from build123d import *

# Parameters (mm, degrees)
F1_DEPTH  = 26
F2_DEPTH  = 4
F3_W      = 90
F3_H      = 64
F4_DEPTH  = 2
F6_DEPTH  = 2
F7_R      = 2.5
F8_DEPTH  = 2
F9_R      = 2.5
F10_DEPTH = 2
F11_W     = 5
F11_H     = 50
F11_W_2   = 76
F11_H_2   = 5
F12_DEPTH = 22
F13_R     = 1
F14_DEPTH = 5
F15_R     = 11
F15_R_2   = 5
F16_DEPTH = 2
F17_DEPTH = 5
F19_W     = 20.16
F19_H     = 11.52
F19_R     = 3
F19_R_2   = 2
F20_DEPTH = 5
F19_W_2   = 66
F19_H_2   = 18
F19_R_3   = 1.8
F21_DEPTH = 3
F22_DEPTH = 3
F19_R_4   = 0.8
F23_DEPTH = 1.9
F24_DEPTH = 1.9
F25_DEPTH = 1.9


# Not quite as in the source:
# - a feature names something its author has since deleted; it is built from what else it names


with BuildPart() as f1:
    # F0 (on Top) → F1 (new body)
    with BuildSketch(Plane.XY):
        with BuildLine():
            Line((46, 35), (-46, 35))
            ThreePointArc((-46, 35), (-47.4142135624, 34.4142135624), (-48, 33))
            Line((-48, 33), (-48, -33))
            ThreePointArc((-48, -33), (-47.4142135624, -34.4142135624), (-46, -35))
            Line((-46, -35), (46, -35))
            ThreePointArc((46, -35), (47.4142135624, -34.4142135624), (48, -33))
            Line((48, -33), (48, 33))
            ThreePointArc((48, 33), (47.4142135624, 34.4142135624), (46, 35))
        make_face()
    extrude(amount=F1_DEPTH)


with BuildPart() as f2:
    # F2 (new): a face of the model
    f2_faces = [f1.part.faces().sort_by_distance(p)[0] for p in [
        (0, 0, 26),
    ]]
    extrude(f2_faces, amount=F2_DEPTH)

    # F5 (on face) → F6 (join)
    with BuildSketch(Plane.XY.offset(30)):
        with BuildLine():
            Line((45.25, 33), (-45.25, 33))
            ThreePointArc((-45.25, 33), (-45.7803300859, 32.7803300859), (-46, 32.25))
            Line((-46, 32.25), (-46, -32.25))
            ThreePointArc((-46, -32.25), (-45.7803300859, -32.7803300859), (-45.25, -33))
            Line((-45.25, -33), (45.25, -33))
            ThreePointArc((45.25, -33), (45.7803300859, -32.7803300859), (46, -32.25))
            Line((46, -32.25), (46, 32.25))
            ThreePointArc((46, 32.25), (45.7803300859, 32.7803300859), (45.25, 33))
        make_face()
        with BuildLine():
            ThreePointArc((-45.25, 32), (-45.1767766953, 32.1767766953), (-45, 32.25))
            Line((-45, 32.25), (45, 32.25))
            ThreePointArc((45, 32.25), (45.1767766953, 32.1767766953), (45.25, 32))
            Line((45.25, 32), (45.25, -32))
            ThreePointArc((45.25, -32), (45.1767766953, -32.1767766953), (45, -32.25))
            Line((45, -32.25), (-45, -32.25))
            ThreePointArc((-45, -32.25), (-45.1767766953, -32.1767766953), (-45.25, -32))
            Line((-45.25, -32), (-45.25, 32))
        make_face(mode=Mode.SUBTRACT)
    extrude(amount=F6_DEPTH)

    # F9 (on face) → F10 (cut)
    with BuildSketch(Plane.XY.offset(30)):
        with Locations((-41.75, -28.75)):
            Circle(F9_R)
        with Locations((-41.75, 28.75)):
            Circle(F9_R)
        with Locations((41.75, 28.75)):
            Circle(F9_R)
        with Locations((41.75, -28.75)):
            Circle(F9_R)
    extrude(amount=-F10_DEPTH, mode=Mode.SUBTRACT)


with BuildPart() as f1_1:
    add(f1.part)

    # F3 (on face) → F4 (cut)
    with BuildSketch(Plane.XY.offset(26)):
        with BuildLine():
            Line((45, 33), (-45, 33))
            ThreePointArc((-45, 33), (-45.7071067812, 32.7071067812), (-46, 32))
            Line((-46, 32), (-46, -32))
            ThreePointArc((-46, -32), (-45.7071067812, -32.7071067812), (-45, -33))
            Line((-45, -33), (45, -33))
            ThreePointArc((45, -33), (45.7071067812, -32.7071067812), (46, -32))
            Line((46, -32), (46, 32))
            ThreePointArc((46, 32), (45.7071067812, 32.7071067812), (45, 33))
        make_face()
        Rectangle(F3_W, F3_H, mode=Mode.SUBTRACT)
    extrude(amount=-F4_DEPTH, mode=Mode.SUBTRACT)

    # F7 (on face) → F8 (cut)
    with BuildSketch(Plane.XY.offset(26)):
        with Locations((-41.5, -28.5)):
            Circle(F7_R)
        with Locations((-41.4999984205, 28.5)):
            Circle(F7_R)
        with Locations((41.5, 28.5)):
            Circle(F7_R)
        with Locations((41.5, -28.5)):
            Circle(F7_R)
    extrude(amount=-F8_DEPTH, mode=Mode.SUBTRACT)

    # F11 (on face) → F12 (cut)
    with BuildSketch(Plane.XY.offset(26)):
        with Locations((-40.5, 0)):
            Rectangle(F11_W, F11_H)
        with Locations((0, -27.5)):
            Rectangle(F11_W_2, F11_H_2)
        Rectangle(F11_W_2, F11_H)
        with Locations((0, 27.5)):
            Rectangle(F11_W_2, F11_H_2)
        with Locations((40.5, 0)):
            Rectangle(F11_W, F11_H)
    extrude(amount=-F12_DEPTH, mode=Mode.SUBTRACT)

    # F13 (on face) → F14 (cut, through all)
    with BuildSketch(Plane.YZ.offset(48)):
        with Locations((7.9999985173, 14.5000000224)):
            Circle(F13_R)
        with Locations((7.9999985173, 11.5000000224)):
            Circle(F13_R)
        with Locations((10.9999985173, 11.5000000224)):
            Circle(F13_R)
        with Locations((10.9999985173, 14.5000000224)):
            Circle(F13_R)
        with Locations((13.9999985173, 14.5000000224)):
            Circle(F13_R)
        with Locations((13.9999985173, 11.5000000224)):
            Circle(F13_R)
    extrude(amount=-F14_DEPTH, mode=Mode.SUBTRACT)

    # F15 (on face) → F16 (cut)
    with BuildSketch(Plane(origin=(-48, 0, 0), x_dir=(0, -1, 0), z_dir=(-1, 0, 0))):
        with Locations((6.9999988191, 12.5000002682)):
            Circle(F15_R)
        with Locations((6.9999988191, 12.5000002682)):
            Circle(F15_R_2, mode=Mode.SUBTRACT)
    extrude(amount=-F16_DEPTH, mode=Mode.SUBTRACT)

    # F15 (on face) → F17 (cut, through all)
    with BuildSketch(Plane(origin=(-48, 0, 0), x_dir=(0, -1, 0), z_dir=(-1, 0, 0))):
        with Locations((6.9999988191, 12.5000002682)):
            Circle(F15_R_2)
    extrude(amount=-F17_DEPTH, mode=Mode.SUBTRACT)

    # F19 (on face) → F20 (cut, through all)
    with BuildSketch(Plane(origin=(0, -30, 0), x_dir=(-1, 0, 0), z_dir=(0, 1, 0))):
        with Locations((4.7299169147, 14.0678631142)):
            Rectangle(F19_W, F19_H)
        with Locations((28.8399169147, 14.0678631142)):
            Circle(F19_R)
        with Locations((-11.1500830853, 14.0678631142)):
            Circle(F19_R_2)
        with Locations((-17.7100830853, 14.0678631142)):
            Circle(F19_R_2)
        with Locations((-24.2600830853, 14.0678631142)):
            Circle(F19_R_2)
        with BuildLine():
            ThreePointArc((-30.8900830853, 11.0678631142), (-30.5971898665, 10.360756333), (-29.8900830853, 10.0678631142))
            Line((-29.8900830853, 10.0678631142), (-28.9900830853, 10.0678631142))
            ThreePointArc((-28.9900830853, 10.0678631142), (-28.2829763041, 10.360756333), (-27.9900830853, 11.0678631142))
            Line((-27.9900830853, 11.0678631142), (-27.9900830853, 17.0678631142))
            ThreePointArc((-27.9900830853, 17.0678631142), (-28.2829763041, 17.7749698954), (-28.9900830853, 18.0678631142))
            Line((-28.9900830853, 18.0678631142), (-29.8900830853, 18.0678631142))
            ThreePointArc((-29.8900830853, 18.0678631142), (-30.5971898665, 17.7749698954), (-30.8900830853, 17.0678631142))
            Line((-30.8900830853, 17.0678631142), (-30.8900830853, 11.0678631142))
        make_face()
    extrude(amount=-F20_DEPTH, mode=Mode.SUBTRACT)

    # F19 (on face) → F21 (cut)
    with BuildSketch(Plane(origin=(0, -30, 0), x_dir=(-1, 0, 0), z_dir=(0, 1, 0))):
        with Locations((-0.1600830853, 14.0678631142)):
            Rectangle(F19_W_2, F19_H_2)
        with Locations((-24.0000830853, 7.5678631142)):
            Circle(F19_R_3, mode=Mode.SUBTRACT)
        with BuildLine():
            Line((-28.9900830853, 10.0678631142), (-29.8900830853, 10.0678631142))
            ThreePointArc((-29.8900830853, 10.0678631142), (-30.5971898665, 10.360756333), (-30.8900830853, 11.0678631142))
            Line((-30.8900830853, 11.0678631142), (-30.8900830853, 17.0678631142))
            ThreePointArc((-30.8900830853, 17.0678631142), (-30.5971898665, 17.7749698954), (-29.8900830853, 18.0678631142))
            Line((-29.8900830853, 18.0678631142), (-28.9900830853, 18.0678631142))
            ThreePointArc((-28.9900830853, 18.0678631142), (-28.2829763041, 17.7749698954), (-27.9900830853, 17.0678631142))
            Line((-27.9900830853, 17.0678631142), (-27.9900830853, 11.0678631142))
            ThreePointArc((-27.9900830853, 11.0678631142), (-28.2829763041, 10.360756333), (-28.9900830853, 10.0678631142))
        make_face(mode=Mode.SUBTRACT)
        with Locations((-24.2600830853, 14.0678631142)):
            Circle(F19_R_2, mode=Mode.SUBTRACT)
        with Locations((-17.7100830853, 14.0678631142)):
            Circle(F19_R_2, mode=Mode.SUBTRACT)
        with Locations((-11.1500830853, 14.0678631142)):
            Circle(F19_R_2, mode=Mode.SUBTRACT)
        with Locations((30.1799169147, 7.5678631142)):
            Circle(F19_R_3, mode=Mode.SUBTRACT)
        with Locations((4.7299169147, 14.0678631142)):
            Rectangle(F19_W, F19_H, mode=Mode.SUBTRACT)
        with Locations((28.8399169147, 14.0678631142)):
            Circle(F19_R, mode=Mode.SUBTRACT)
        with Locations((30.1799169147, 20.5678631142)):
            Circle(F19_R_3, mode=Mode.SUBTRACT)
    extrude(amount=F21_DEPTH, mode=Mode.SUBTRACT)

    # F19 (on face) → F22 (cut)
    with BuildSketch(Plane(origin=(0, -30, 0), x_dir=(-1, 0, 0), z_dir=(0, 1, 0))):
        with Locations((-0.1600830853, 14.0678631142)):
            Rectangle(F19_W_2, F19_H_2)
        with Locations((-24.0000830853, 7.5678631142)):
            Circle(F19_R_3, mode=Mode.SUBTRACT)
        with BuildLine():
            Line((-28.9900830853, 10.0678631142), (-29.8900830853, 10.0678631142))
            ThreePointArc((-29.8900830853, 10.0678631142), (-30.5971898665, 10.360756333), (-30.8900830853, 11.0678631142))
            Line((-30.8900830853, 11.0678631142), (-30.8900830853, 17.0678631142))
            ThreePointArc((-30.8900830853, 17.0678631142), (-30.5971898665, 17.7749698954), (-29.8900830853, 18.0678631142))
            Line((-29.8900830853, 18.0678631142), (-28.9900830853, 18.0678631142))
            ThreePointArc((-28.9900830853, 18.0678631142), (-28.2829763041, 17.7749698954), (-27.9900830853, 17.0678631142))
            Line((-27.9900830853, 17.0678631142), (-27.9900830853, 11.0678631142))
            ThreePointArc((-27.9900830853, 11.0678631142), (-28.2829763041, 10.360756333), (-28.9900830853, 10.0678631142))
        make_face(mode=Mode.SUBTRACT)
        with Locations((-24.2600830853, 14.0678631142)):
            Circle(F19_R_2, mode=Mode.SUBTRACT)
        with Locations((-17.7100830853, 14.0678631142)):
            Circle(F19_R_2, mode=Mode.SUBTRACT)
        with Locations((-11.1500830853, 14.0678631142)):
            Circle(F19_R_2, mode=Mode.SUBTRACT)
        with Locations((30.1799169147, 7.5678631142)):
            Circle(F19_R_3, mode=Mode.SUBTRACT)
        with Locations((4.7299169147, 14.0678631142)):
            Rectangle(F19_W, F19_H, mode=Mode.SUBTRACT)
        with Locations((28.8399169147, 14.0678631142)):
            Circle(F19_R, mode=Mode.SUBTRACT)
        with Locations((30.1799169147, 20.5678631142)):
            Circle(F19_R_3, mode=Mode.SUBTRACT)
    extrude(amount=-F22_DEPTH, mode=Mode.SUBTRACT)

    # F19 (on face) → F23 (join)
    with BuildSketch(Plane(origin=(0, -30, 0), x_dir=(-1, 0, 0), z_dir=(0, 1, 0))):
        with Locations((30.1799169147, 20.5678631142)):
            Circle(F19_R_3)
        with Locations((30.1799169147, 20.5678631142)):
            Circle(F19_R_4, mode=Mode.SUBTRACT)
    extrude(amount=F23_DEPTH)

    # F19 (on face) → F24 (join)
    with BuildSketch(Plane(origin=(0, -30, 0), x_dir=(-1, 0, 0), z_dir=(0, 1, 0))):
        with Locations((30.1799169147, 7.5678631142)):
            Circle(F19_R_3)
        with Locations((30.1799169147, 7.5678631142)):
            Circle(F19_R_4, mode=Mode.SUBTRACT)
    extrude(amount=F24_DEPTH)

    # F19 (on face) → F25 (join)
    with BuildSketch(Plane(origin=(0, -30, 0), x_dir=(-1, 0, 0), z_dir=(0, 1, 0))):
        with Locations((-24.0000830853, 7.5678631142)):
            Circle(F19_R_3)
        with Locations((-24.0000830853, 7.5678631142)):
            Circle(F19_R_4, mode=Mode.SUBTRACT)
    extrude(amount=F25_DEPTH)


with BuildPart() as f27_1:
    # F27: copy of F2
    add(f2.part)


with BuildPart() as f29_1:
    # F29: copy of F2
    add(f2.part)


solid = f2.part
Geometry check sheet. Reference: the model listing, model coordinates, mm. A direction names the side the tool comes from. Round coordinates to 2 decimals unless told otherwise and drop trailing zeros. Loops run counter-clockwise (first coordinate to the right, second up) from the corner with the lowest first, then second, coordinate; pieces in that order, holes last.
Item 1: Gauge pin test, flat ends, axial feed: pin 1 (0.6 mm diameter, centred on y = 2.5, z = 31, fed in from -X); pin 2 (2.5 mm diameter, centred on x = -42.5, y = -29, fed in from +Z); pin 3 (1 mm diameter, centred on x = -3, z = 31, fed in from -Y). Record the tip position at first contact, or that the pin passes through.
Item 2: Access from +Z, -Z, +X, -X, +Y, -Y to the whole of each face (thin tool, end or side, straight path). Record for faces 4 (the flat face through (-46, 0, 31)), 5 (the flat face through (-1, -35, 28)), 6 (the flat face through (1, 33, 31)), 7 (the flat face through (46, 0, 31)), 8 (the cylindrical face through (43.09, 30.86, 29.01)).
Item 3: Cross-section at A-A on x = -38. Record the boundary of the cut face in (y, z), then the cut area to 3 significant figures.
Item 4: Thickness scan on line 1 (Y direction, x = 41.75, z = 28.9); line 2 (X direction, y = 14, z = 30.75); line 3 (Y direction, x = 28, z = 30.8). Record the ranges inside material, lowest first.
Item 5: Cross-section at C-C on x = 40.5. Record the boundary of the cut face in (y, z), then the cut area to 3 significant figures.
Item 6: Cross-section at B-B on y = 22. Record the boundary of the cut face in (x, z).
Item 7: Mould release check, pull along X, two halves, no side actions. Record for faces 1 (the cylindrical face through (-47.4, 34.43, 27.97)), 2 (the flat face through (1, -32.25, 31)), 3 (the flat face through (-1, 0, 26)): pulls with the +X half, pulls with the -X half, needs draft (parallel to the pull), parting line crosses it, or undercut.
Answer sheet:
1. pin 1: stops at x = -46
1. pin 2: stops at z = 28
1. pin 3: stops at y = -33
2. face 4: +Z, -X, +Y, -Y
2. face 5: +Z, -Z, +X, -X, -Y
2. face 6: +Z, +X, -X, +Y
2. face 7: +Z, +X, +Y, -Y
2. face 8: +Z
3. outline: (-35, 26) - (35, 26) - (35, 30) - (33, 30) - (33, 32) - (32.25, 32) - (32.25, 30) - (-32.25, 30) - (-32.25, 32) - (-33, 32) - (-33, 30) - (-35, 30) - close
3. area: 283 mm2
4. line 1: y = -35 to -31.25, -26.25 to 26.25, 31.25 to 35
4. line 2: x = -46 to -45.25, 45.25 to 46
4. line 3: y = -33 to -32.25, 32.25 to 33
5. outline: (-35, 26) - (35, 26) - (35, 30) - (33, 30) - (33, 32) - (32.25, 32) - (32.25, 30) - (30.92, 30) - (30.92, 28) - (26.58, 28) - (26.58, 30) - (-26.58, 30) - (-26.58, 28) - (-30.92, 28) - (-30.92, 30) - (-32.25, 30) - (-32.25, 32) - (-33, 32) - (-33, 30) - (-35, 30) - close
5. area: 266 mm2
6. outline: (-48, 26) - (48, 26) - (48, 30) - (46, 30) - (46, 32) - (45.25, 32) - (45.25, 30) - (-45.25, 30) - (-45.25, 32) - (-46, 32) - (-46, 30) - (-48, 30) - close
7. face 1: pulls with the -X half
7. face 2: undercut
7. face 3: needs draft
